```python
from build123d import *

# Parameters (mm, degrees)
SKETCH16_W          = 60.3
SKETCH16_H          = 58.8
SKETCH16_R          = 22
BOSS_EXTRUDE2_DEPTH = 5
SKETCH22_W          = 60.3
SKETCH22_H          = 2.5
BOSS_EXTRUDE7_DEPTH = 50
SKETCH23_R          = 26
SKETCH23_R_2        = 22
BOSS_EXTRUDE8_DEPTH = 5
CUT_EXTRUDE3_DEPTH  = 2.5
BOSS_EXTRUDE9_DEPTH = 2.5


with BuildPart() as part:
    # Sketch16 → Boss-Extrude2 (new body)
    with BuildSketch(Plane.XY):
        with Locations((0, 1.75)):
            Rectangle(SKETCH16_W, SKETCH16_H)
        Circle(SKETCH16_R, mode=Mode.SUBTRACT)
    extrude(amount=-BOSS_EXTRUDE2_DEPTH)

    # Sketch22 → Boss-Extrude7 (add)
    with BuildSketch(Plane(origin=(0, 31.15, 0), x_dir=(1, 0, 0), z_dir=(0, 1, 0))):
        with Locations((0, 3.75)):
            Rectangle(SKETCH22_W, SKETCH22_H)
    extrude(amount=-BOSS_EXTRUDE7_DEPTH)

    # Sketch23 → Boss-Extrude8 (add)
    with BuildSketch(Plane.XY):
        with Locations((0.443922204, 0)):
            Circle(SKETCH23_R)
        Circle(SKETCH23_R_2, mode=Mode.SUBTRACT)
    extrude(amount=BOSS_EXTRUDE8_DEPTH)

    # Sketch24 → Cut-Extrude3 (cut)
    with BuildSketch(Plane.XY.offset(-2.5)):
        with BuildLine():
            Line((-11.343610536, -18.85), (11.343610536, -18.85))
            ThreePointArc((11.343610536, -18.85), (0, -7.506389464), (-11.343610536, -18.85))
        make_face()
    extrude(amount=-CUT_EXTRUDE3_DEPTH, mode=Mode.SUBTRACT)

    # Sketch25 → Boss-Extrude9 (add)
    with BuildSketch(Plane.XY.offset(-2.5)):
        with BuildLine():
            Line((11.343610536, -18.85), (-11.343610536, -18.85))
            ThreePointArc((-11.343610536, -18.85), (0, -22), (11.343610536, -18.85))
        make_face()
    extrude(amount=-BOSS_EXTRUDE9_DEPTH)


solid = part.part
```
The model under review builds one solid part; all positions refer to its coordinate system, in mm. A direction names the side the tool comes from. Round coordinates to 2 decimals unless told otherwise and drop trailing zeros. Order: outer loops, then holes, each group sorted by start corner. A loop starts at its lowest first (then second) coordinate and runs counter-clockwise, first axis right, second up. Notation, with made-up numbers: M 19,73.5 L 23,73.5 A20 cw 23,91.5 Z; hole C -4,58 d5. An arc over 180 degrees is marked long. Use a Markdown table: item, result.
1) Consider section D-D (x = 17.5). Write out the cut boundary in (y, z), then the cut area to 3 significant figures.
Report:
| item | result |
|---|---|
| outline | M -27.65,-5 L 31.15,-5 L 31.15,0 L 19.62,0 L 19.62,5 L 13.33,5 L 13.33,-2.5 L -13.33,-2.5 L -13.33,5 L -19.62,5 L -19.62,0 L -27.65,0 Z |
| area | 290 mm^2 |
2) Draft analysis for pull direction Y (two halves, no side actions). For faces 4 (the face through (-5.192, -25.382, 2.465)), 5 (the face through (0, -18.85, -4)), 6 (the face through (30.15, 1, -2)), state which applies: released by +Y, released by -Y, zero draft, split by the parting line, or undercut.
Report:
| item | result |
|---|---|
| face 4 | split by the parting line |
| face 5 | undercut |
| face 6 | zero draft |
3) Tool access review of faces 1 (the face through (0, -20, -2.5)), 2 (the face through (0.25, -7.51, -3.73)), 3 (the face through (0, -27.65, -2)): name each direction out of +Z, -Z, +X, -X, +Y, -Y from which nothing blocks a thin tool from reaching the whole face with its end or side.
Report:
| item | result |
|---|---|
| face 1 | +Z |
| face 2 | +Z, -Z |
| face 3 | +Z, -Z, +X, -X, -Y |
4) Consider section C-C (z = -1). Write out the cut boundary in (x, y), then the cut area to 3 significant figures.
Report:
| item | result |
|---|---|
| outline | M -30.15,-27.65 L 30.15,-27.65 L 30.15,31.15 L -30.15,31.15 Z; hole C 0,0 d44 |
| area | 2,030 mm^2 |
5) Wall thickness on line 1 along Y through (x, z) = (0, 1.65); line 2 along Z through (x, y) = (-3.5, -20); line 3 along X through (y, z) = (0, -1.7): over which ranges is each line inside the solid? List them lowest first. Write a range as [from, to].
Report:
| item | result |
|---|---|
| line 1 | [-26, -22], [22, 26] |
| line 2 | [-5, -2.5] |
| line 3 | [-30.15, -22], [22, 30.15] |
6) Insertion check: pin 1 (4 mm diameter, centred on y = 11, z = 0.5, fed in from -X); pin 2 (2.5 mm diameter, centred on x = 1, y = -20.5, fed in from +Z). Each pin has a flat end and moves straight along its axis. Give the tip position at first contact, or say it passes through.
Report:
| item | result |
|---|---|
| pin 1 | x = -30.15 |
| pin 2 | z = -2.5 |
7) Consider section A-A (x = 0). Write out the cut boundary in (y, z), then the cut area to 3 significant figures.
Report:
| item | result |
|---|---|
| outline | M -27.65,-5 L -18.85,-5 L -18.85,-2.5 L -22,-2.5 L -22,5 L -26,5 L -26,0 L -27.65,0 Z; M -7.51,-5 L 31.15,-5 L 31.15,0 L 26,0 L 26,5 L 22,5 L 22,-2.5 L -7.51,-2.5 Z |
| area | 196 mm^2 |
8) Consider section B-B (y = 0). Write out the cut boundary in (x, z), then the cut area to 4 significant figures.
Report:
| item | result |
|---|---|
| outline | M -30.15,-5 L 30.15,-5 L 30.15,0 L 26.44,0 L 26.44,5 L 22,5 L 22,-2.5 L -22,-2.5 L -22,5 L -25.56,5 L -25.56,0 L -30.15,0 Z |
| area | 231.5 mm^2 |
